Geometry check sheet. Reference: the model listing, model coordinates, mm. Face numbers are marked on the shaded views. A direction names the side the tool comes from. Round coordinates to 2 decimals unless told otherwise and drop trailing zeros. Write each loop counter-clockwise with the first axis right and the second up, starting at its lowest first coordinate (ties: lowest second). Pieces come first, ordered by that corner, then holes. Notation, with made-up numbers: (44, 4) -> (93, 4) arc R24 ccw to (93, 33) -> close; hole circle Ø8 at (-25.75, 44.5). An arc over 180 degrees is marked (long way). Use a Markdown table: item, result.
Autodesk Inventor part; units mm, degrees
ref_plane "YZ Plane" through (0, 0, 0) normal (1, 0, 0) x (0, 1, 0)
ref_plane "XZ Plane" through (0, 0, 0) normal (0, 1, 0) x (-1, 0, 0)
ref_plane "XY Plane" through (0, 0, 0) normal (0, 0, 1) x (1, 0, 0)
sketch "Sketch1" plane through (0, 0, 0) normal (0, 0, 1) x (1, 0, 0)
  line L0 (0, 0) -> (0, 20)
  line L1 (0, 0) -> (32, 0)
  line L2 (32, 0) -> (0, 20)
  dimension "d0" = 20
  dimension "d1" = 32
extrude "Extrusion1" add sketch "Sketch1" along normal blind 47
sketch "Sketch2" plane through (0, 0, 0) normal (-1, 0, 0) x (0, 0, 1)
  line L0 (0, 0) -> (47, 0)
  line L1 (0, 20) -> (0, 0)
  line L2 (0, 0) -> (0, 20)
  line L3 (0, 20) -> (47, 20)
  line L4 (0, 20) -> (47, 20)
  line L5 (23.5, 13) -> (16.5, 13)
  line L6 (16.5, 13) -> (30.5078, 13)
  line L7 (30.5078, 13) -> (30.5078, 6.9967)
  line L8 (30.5078, 6.9967) -> (16.5, 6.9967)
  line L9 (16.5, 6.9967) -> (16.5, 13)
  dimension "d5" = 7
  dimension "d6" = 15.24
extrude "Extrusion2" cut sketch "Sketch2" against normal blind 19
properties part number "mouseBottom"
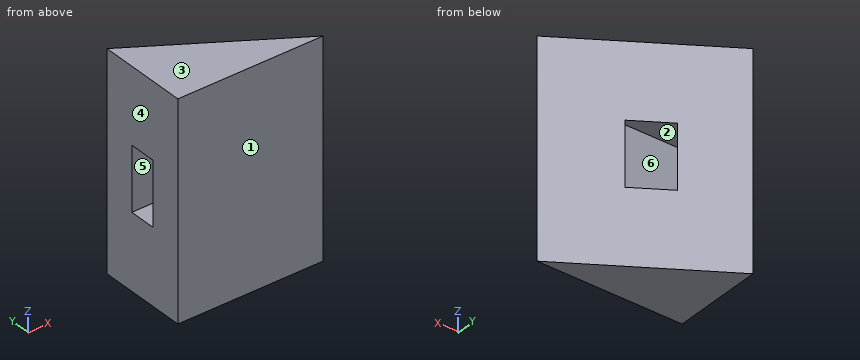
(1) Section check A-A on y = 11.75. Record the cut outline in (x, z).
A:
| item | result |
|---|---|
| outline | (0, 0) -> (13.2, 0) -> (13.2, 16.5) -> (0, 16.5) -> close; (0, 30.51) -> (13.2, 30.51) -> (13.2, 47) -> (0, 47) -> close |
(2) Section check D-D on y = 4.75. Record the cut outline in (x, z).
A:
| item | result |
|---|---|
| outline | (0, 0) -> (24.4, 0) -> (24.4, 47) -> (0, 47) -> close |
(3) Release check for a two-part mould opening along Z. For the marked faces 3, 4, 5 and 6 record: +Z half, -Z half, draft (parallel to the pull), parting line (faces both ways), or undercut.
A:
| item | result |
|---|---|
| face 3 | +Z half |
| face 4 | draft |
| face 5 | undercut |
| face 6 | undercut |
(4) Section check C-C on x = 18. Record the cut outline in (y, z).
A:
| item | result |
|---|---|
| outline | (0, 0) -> (8.75, 0) -> (8.75, 16.5) -> (7, 16.5) -> (7, 30.51) -> (8.75, 30.51) -> (8.75, 47) -> (0, 47) -> close |
(5) Section check B-B on z = 23.5. Record the cut outline in (x, y) (3 decimals).
A:
| item | result |
|---|---|
| outline | (0, 0) -> (32, 0) -> (19, 8.125) -> (19, 6.997) -> (0, 6.997) -> close; (0, 13) -> (11.2, 13) -> (0, 20) -> close |
(6) Thickness scan on line 1 (Z direction, x = 2, y = 11.25); line 2 (Y direction, x = 2.5, z = 22); line 3 (Y direction, x = 7.5, z = 31.5). Record the ranges inside material, lowest first.
A:
| item | result |
|---|---|
| line 1 | z = 0 to 16.5, 30.51 to 47 |
| line 2 | y = 0 to 7, 13 to 18.44 |
| line 3 | y = 0 to 15.31 |
(7) Access from +Z, -Z, +X, -X, +Y, -Y to the whole of each face (thin tool, end or side, straight path). Record for the marked faces 1 and 2.
A:
| item | result |
|---|---|
| face 1 | +Z, -Z, +X, -X, -Y |
| face 2 | -X |
(8) Gauge pin test, flat ends, axial feed: pin 1 Ø1.5 at (x, z) = (15, 28.5) entering from +Y; pin 2 Ø1.2 at (y, z) = (8, 23.5) entering from -X; pin 3 Ø15.5 at (x, z) = (13.5, 20) entering from +Y. Record the tip position at first contact, or that the pin passes through.
A:
| item | result |
|---|---|
| pin 1 | stops at y = 7 |
| pin 2 | stops at x = 19 |
| pin 3 | stops at y = 16.41 |
